The model under review builds one solid part; all positions refer to its coordinate system, in mm. Face numbers are marked on the shaded views. A direction names the side the tool comes from. Coordinates: 2 decimals unless noted, no trailing zeros. Loops run counter-clockwise (first coordinate to the right, second up) from the corner with the lowest first, then second, coordinate; pieces in that order, holes last. Notation, with made-up numbers: M 65.25,-17.5 L 93.25,-17.5 A20 ccw 93.25,9.5 Z; hole C 33,79.5 d5. An arc over 180 degrees is marked long. Use one line per item in the form item = value.
```python
from build123d import *

# Parameters (mm, degrees)
SKETCH1_R          = 0.6
CUT_EXTRUDE1_DEPTH = 2
CIRPATTERN1_COUNT  = 4


with BuildPart() as part:
    # Esquisse1 → Révolution1 (revolve)
    with BuildSketch(Plane.XY):
        Polygon((2.75, 0), (2.75, 3), (1.5, 3), (1.5, 4), (3, 4), (3, 5), (3.75, 5), (3.75, 4.5), (10, 4.5), (10, 2.5), (4.5, 2.5), (4.5, 0), align=None)
    revolve(axis=Axis((0, 0, 0), (0, 1, 0)))

    # Sketch1 → Cut-Extrude1 (cut)
    with BuildSketch(Plane(origin=(0, 4.5, 0), x_dir=(1, 0, 0), z_dir=(0, 1, 0))):
        with Locations((0, 7.5)):
            Circle(SKETCH1_R)
        with Locations((3, 7.5)):
            Circle(SKETCH1_R)
        with Locations((-3, 7.5)):
            Circle(SKETCH1_R)
    cut_extrude1 = extrude(amount=-CUT_EXTRUDE1_DEPTH, mode=Mode.SUBTRACT)

    # CirPattern1: Cut-Extrude1 ×4 about axis
    cirpattern1_axis = Axis((0, 0, 0), (0, 1, 0))
    for i in range(1, CIRPATTERN1_COUNT):
        add(cut_extrude1.rotate(cirpattern1_axis, i * 360 / CIRPATTERN1_COUNT), mode=Mode.SUBTRACT)


solid = part.part
```
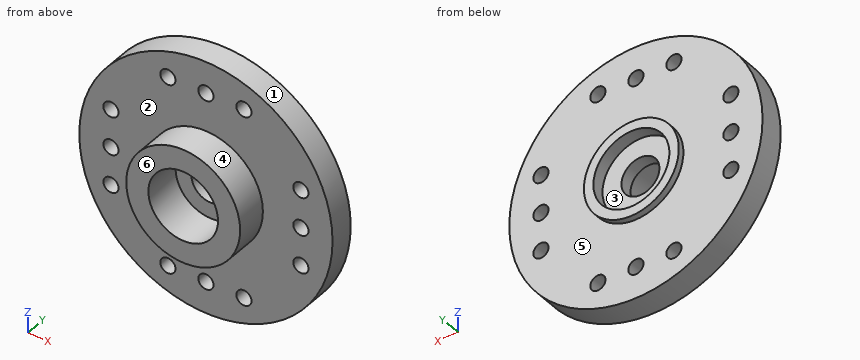
1. Insertion check: P1, Ø0.7, axis at x = 7.5, z = -3, coming from the +Y side; P2, Ø1.6, axis at x = 3, z = -7.5, coming from the -Y side; P3, Ø3, axis at y = 4.5, z = 3.5, coming from the -X side; P4, Ø1.4, axis at x = 3, z = 7.5, coming from the +Y side. Each pin has a flat end and moves straight along its axis. Give the tip position at first contact, or say it passes through.
Response values:
P1 = through
P2 = 2.5
P3 = -9.8
P4 = 4.5
2. Wall thickness on line 1 along X through (y, z) = (3.05, 0); line 2 along X through (y, z) = (4.1, 0); line 3 along Z through (x, y) = (-3, 3.15): over which ranges is each line inside the solid? List them lowest first. Write a range as from..to.
Response values:
line_1 = -10..-8.1, -6.9..-1.5, 1.5..6.9, 8.1..10
line_2 = -10..-8.1, -6.9..-3, 3..6.9, 8.1..10
line_3 = -9.54..-8.1, -6.9..6.9, 8.1..9.54
3. The part is to be moulded in two halves that separate along Z. For the marked faces 1, 2 and 3, say which applies: pulls with the +Z half, pulls with the -Z half, needs draft (parallel to the pull), parting line crosses it, or undercut.
Response values:
face_1 = parting line crosses it
face_2 = needs draft
face_3 = undercut
4. Machinability: for the marked faces 4, 5 and 6, which of the approach directions +Z, -Z, +X, -X, +Y, -Y give a long, thin tool a straight path to every point of the face, cutting with its end or side? Answer none if there is none.
Response values:
face_4 = -Y
face_5 = +Y
face_6 = +Z, -Z, +X, -X, -Y
5. Add section A-A (z = 0). Count the separate pieces of the cut face and the enclosed holes in it, then the cut area to 4 significant figures.
Response values:
separate_pieces = 4
enclosed_holes = 0
area = 35.95 mm^2
6. Add section D-D (y = 0.5). State the section outline as (x, z) points.
Response values:
outline = C 0,0 d9; hole C 0,0 d5.5
